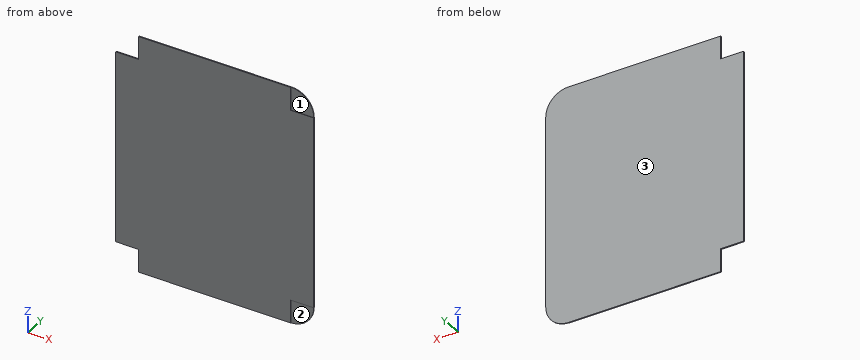
```python
from build123d import *

# Parameters (mm, degrees)
EXTRUDE_1_DEPTH = 3
EXTRUDE_2_DEPTH = 2


with BuildPart() as part:
    # 草图1 → 凸台-拉伸1 (new body)
    with BuildSketch(Plane(origin=(0, 0, 0), x_dir=(1, 0, 0), z_dir=(0, 1, 0))):
        Polygon((-240.917431193, -196.788990826), (-240.917431193, -256.788990826), (159.082568807, -256.788990826), (159.082568807, -196.788990826), (219.082568807, -196.788990826), (219.082568807, 303.211009174), (159.082568807, 303.211009174), (159.082568807, 363.211009174), (-240.917431193, 363.211009174), (-240.917431193, 303.211009174), (-300.917431193, 303.211009174), (-300.917431193, -196.788990826), align=None)
    extrude(amount=EXTRUDE_1_DEPTH)

    # 草图2 → 凸台-拉伸2 (add)
    with BuildSketch(Plane(origin=(0, 3, 0), x_dir=(1, 0, 0), z_dir=(0, 1, 0))):
        with BuildLine():
            Line((159.082568807, 303.211009174), (219.082568807, 303.211009174))
            ThreePointArc((219.082568807, 303.211009174), (201.508975679, 345.637416046), (159.082568807, 363.211009174))
            Line((159.082568807, 363.211009174), (159.082568807, 303.211009174))
        make_face()
        with BuildLine():
            Line((159.082568807, -256.788990826), (159.082568807, -196.788990826))
            Line((159.082568807, -196.788990826), (219.082568807, -196.788990826))
            ThreePointArc((219.082568807, -196.788990826), (201.508975679, -239.215397697), (159.082568807, -256.788990826))
        make_face()
    extrude(amount=-EXTRUDE_2_DEPTH)


solid = part.part
```
Work out the finished part from the listing and answer in its coordinate system (mm). Face numbers are marked on the shaded views. A direction names the side the tool comes from. Round coordinates to 2 decimals unless told otherwise and drop trailing zeros. Loops run counter-clockwise (first coordinate to the right, second up) from the corner with the lowest first, then second, coordinate; pieces in that order, holes last.
(1) The part is cut by section A-A, the plane y = 2.35. Give the vertices of the cut face in (x, z), and give its area (3 significant figures).
Computed values:
outline: (-300.92, -303.21) - (-240.92, -303.21) - (-240.92, -363.21) - (159.08, -363.21) arc R60 ccw to (219.08, -303.21) - (219.08, 196.79) arc R60 ccw to (159.08, 256.79) - (-240.92, 256.79) - (-240.92, 196.79) - (-300.92, 196.79) - close
area: 314,000 mm2
(2) The part is cut by section B-B, the plane z = -316. Give the vertices of the cut face in (x, y).
Computed values:
outline: (-240.92, 0) - (159.08, 0) - (159.08, 1) - (217.7, 1) - (217.7, 3) - (-240.92, 3) - close
(3) Each of these flat-tipped pins is pushed along its axis until it touches: P1, Ø0.9, axis at x = -279, y = 1.5, coming from the +Z side; P2, Ø1.1, axis at x = 175, y = 0.5, coming from the +Z side; P3, Ø1.5, axis at x = -284, y = 1, coming from the -Z side. Where does it stop, or does it pass through?
Computed values:
P1: stops at z = 196.79
P2: stops at z = 254.7
P3: stops at z = -303.21
(4) Find the intervals of material crossed by L1, parallel to Z at x = -278, y = 0.4, in increasing order.
Computed values:
L1: z = -303.21 to 196.79
(5) For the marked faces 1, 2 and 3, determine the directions among +Z, -Z, +X, -X, +Y, -Y from which every point of the face is accessible in a straight line to the end or side of a thin tool.
Computed values:
face 1: +Z, +X, -Y
face 2: -Z, +X, -Y
face 3: +Z, -Z, +X, -X, +Y
(6) The part is cut by section C-C, the plane z = 211. Give the vertices of the cut face in (x, y).
Computed values:
outline: (-240.92, 0) - (159.08, 0) - (159.08, 1) - (217.38, 1) - (217.38, 3) - (-240.92, 3) - close
